from build123d import *

# Parameters (mm, degrees)
F0_R     = 7.493
F0_R_2   = 1.651
F1_DEPTH = 1.1938
F2_DEPTH = 1.27
F3_R     = 8.8870084673
F3_R_2   = 7.493
F4_DEPTH = 1.1938


with BuildPart() as f1:
    # F0 (on Front) → F1 (new body)
    with BuildSketch(Plane.XZ):
        Circle(F0_R)
        Circle(F0_R_2, mode=Mode.SUBTRACT)
    extrude(amount=F1_DEPTH)

    # F2 (add): a face of the model
    f2_faces = [f1.faces().sort_by_distance(p)[0] for p in [
        (-7.2810659555, -1.1938, 0),
    ]]
    extrude(f2_faces, amount=F2_DEPTH)

    # F3 (on face) → F4 (join)
    with BuildSketch(Plane.XZ.offset(2.4638)):
        Circle(F3_R)
        Circle(F3_R_2, mode=Mode.SUBTRACT)
    extrude(amount=-F4_DEPTH)


solid = f1.part
Check sheet for the modelled part. Datum: model origin and axes. Units: mm. A direction names the side the tool comes from. Coordinates: 2 decimals unless noted, no trailing zeros. Loops run counter-clockwise (first coordinate to the right, second up) from the corner with the lowest first, then second, coordinate; pieces in that order, holes last. Notation, with made-up numbers: (24, -14.5) -> (49, -14.5) arc R21 cw to (49, 9.5) -> close; hole circle Ø8 at (62, 18). An arc over 180 degrees is marked (long way). Write item = value, one per line. Start each with the question number.
1. Draft check along X on faces 3 (the flat face through (-5, -1.27, -6)), 4 (the cylindrical face through (1.525, -1.215, -0.632)), 5 (the cylindrical face through (-7.05, -1.88, -5.41)). Enter one of: released by +X, released by -X, zero draft, split by the parting line, or undercut.
2. Section check D-D on x = 7. Record the cut outline in (y, z).
3. Section check B-B on x = 0. Record the cut outline in (y, z).
4. Section check C-C on y = -1.9. Record the cut outline in (x, z).
5. Depth check by flat-ended pin: P1, Ø1, axis at x = 5, y = -1, coming from the -Z side; P2, Ø9, axis at x = -2, z = 3.5, coming from the +Y side. Enter the tip coordinate at first touch or a pass-through.
6. Tool access check on faces 1 (the flat face through (2, -2.464, 0)), 2 (the cylindrical face through (-0.98, -0.63, 7.43)). Record the directions out of +Z, -Z, +X, -X, +Y, -Y that give a thin tool (end or side, any length) a straight path to the whole face; none if there is none.
7. Material ranges on line 1 (Z direction, x = 0, y = -1); line 2 (Y direction, x = -5.5, z = -6.25); line 3 (Z direction, x = -1.5, y = -1.5), recorded low to high.
8. Section check A-A on z = 0. Record the cut outline in (x, y), then the cut area to 3 significant figures.
Responses:
q1.face_3 = zero draft
q1.face_4 = undercut
q1.face_5 = split by the parting line
q2.outline = (-2.46, -5.48) -> (-1.27, -5.48) -> (-1.27, -2.67) -> (0, -2.67) -> (0, 2.67) -> (-1.27, 2.67) -> (-1.27, 5.48) -> (-2.46, 5.48) -> close
q3.outline = (-2.46, -8.89) -> (-1.27, -8.89) -> (-1.27, -7.49) -> (0, -7.49) -> (0, -1.65) -> (-2.46, -1.65) -> close; (-2.46, 1.65) -> (0, 1.65) -> (0, 7.49) -> (-1.27, 7.49) -> (-1.27, 8.89) -> (-2.46, 8.89) -> close
q4.outline = circle Ø17.77 at (0, 0); hole circle Ø3.3 at (0, 0)
q5.P1 = -7.62
q5.P2 = 0
q6.face_1 = +Z, -Z, +X, -X, -Y
q6.face_2 = +Y
q7.line_1 = -7.49 to -1.65, 1.65 to 7.49
q7.line_2 = -2.46 to -1.27
q7.line_3 = -8.76 to -0.69, 0.69 to 8.76
q8.outline = (-8.89, -2.46) -> (-1.65, -2.46) -> (-1.65, 0) -> (-7.49, 0) -> (-7.49, -1.27) -> (-8.89, -1.27) -> close; (1.65, -2.46) -> (8.89, -2.46) -> (8.89, -1.27) -> (7.49, -1.27) -> (7.49, 0) -> (1.65, 0) -> close
q8.area = 32.1 mm2
